Build history of the part. All positions in model axes, mm. Give positions to 0.01 mm unless a question says otherwise; leave off trailing zeros. Order: outer loops, then holes, each group sorted by start corner. A loop starts at its lowest first (then second) coordinate and runs counter-clockwise, first axis right, second up. Notation, with made-up numbers: (-40, -4) - (9, -4) arc R8 cw to (9, 8) - close; hole circle Ø2 at (80.5, 58.25). An arc over 180 degrees is marked (long way). Use a Markdown table: item, result. Add a question column.
(1) Slice it at D-D (x = 22.5). Write the cut outline in (y, z), then the cut area to 3 significant figures.
(2) Slice it at A-A (y = 0). Write the cut outline in (x, z).
(3) Flat gauge pin, fed straight in: pin 1 (1 mm diameter, centred on y = 1.5, z = 4.5, fed in from -X). Where does the tip first touch, or does it go through?
(4) Mould opens along X. For faces 1 (the face through (-10, 0, 5)), 2 (the face through (3.07, 5.9, 4.93)), 3 (the face through (30, 0, 5)), 4 (the face through (14, -10, 5)) say: +X half, -X half, draft (parallel to the pull), parting line (faces both ways), or undercut.
(5) Wall check: line 1 (Y direction, x = 0, z = 5.25); line 2 (X direction, y = -0.25, z = 4.75); line 3 (Y direction, x = 2, z = 3.25). Give the ranges that are in metal, low to high.
(6) Slice it at B-B (z = 6.75). Write the cut outline in (x, y).
(7) Slice it at C-C (x = 1). Write the cut outline in (y, z).
Autodesk Inventor part; units mm, degrees
ref_plane "YZ Plane" through (0, 0, 0) normal (1, 0, 0) x (0, 1, 0)
ref_plane "XZ Plane" through (0, 0, 0) normal (0, 1, 0) x (-1, 0, 0)
ref_plane "XY Plane" through (0, 0, 0) normal (0, 0, 1) x (1, 0, 0)
sketch "Sketch1" plane through (0, 0, 0) normal (0, 0, 1) x (1, 0, 0)
  circle A0 centre (0, 0) radius 6.65
  arc A1 (0, 10) -> (0, -10) centre (0, 0) ccw
  line L0 (0, 10) -> (30, 10)
  line L1 (30, 10) -> (30, -10)
  line L2 (30, -10) -> (0, -10)
  dimension "d0" = 13.3
  dimension "d2" = 20
  dimension "d3" = 30
  dimension "d4" = 20
extrude "Extrusion1" add sketch "Sketch1" along normal blind 10
fillet "Fillet1" radius 2 10 edges at (30, 10, 5) (30, 0, 10) (-10, 0, 10) (15, -10, 10) (15, 10, 10) (-10, 0, 0) (15, -10, 0) (15, 10, 0) (30, 0, 0) (30, -10, 5)
Solution:
| question | item | result |
|---|---|---|
| 1 | outline | (-10, 2) arc R2 ccw to (-8, 0) - (8, 0) arc R2 ccw to (10, 2) - (10, 8) arc R2 ccw to (8, 10) - (-8, 10) arc R2 ccw to (-10, 8) - close |
| 1 | area | 197 mm2 |
| 2 | outline | (-10, 2) arc R2 ccw to (-8, 0) - (-6.65, 0) - (-6.65, 10) - (-8, 10) arc R2 ccw to (-10, 8) - close; (6.65, 0) - (28, 0) arc R2 ccw to (30, 2) - (30, 8) arc R2 ccw to (28, 10) - (6.65, 10) - close |
| 3 | pin 1 | x = -9.95 |
| 4 | face 1 | -X half |
| 4 | face 2 | undercut |
| 4 | face 3 | +X half |
| 4 | face 4 | draft |
| 5 | line 1 | -10 to -6.65, 6.65 to 10 |
| 5 | line 2 | -10 to -6.65, 6.65 to 30 |
| 5 | line 3 | -10 to -6.34, 6.34 to 10 |
| 6 | outline | (0, -10) - (28, -10) arc R2 ccw to (30, -8) - (30, 8) arc R2 ccw to (28, 10) - (0, 10) arc R10 ccw to start; hole circle Ø13.3 at (0, 0) |
| 7 | outline | (-10, 2) arc R2 ccw to (-8, 0) - (-6.57, 0) - (-6.57, 10) - (-8, 10) arc R2 ccw to (-10, 8) - close; (6.57, 0) - (8, 0) arc R2 ccw to (10, 2) - (10, 8) arc R2 ccw to (8, 10) - (6.57, 10) - close |
